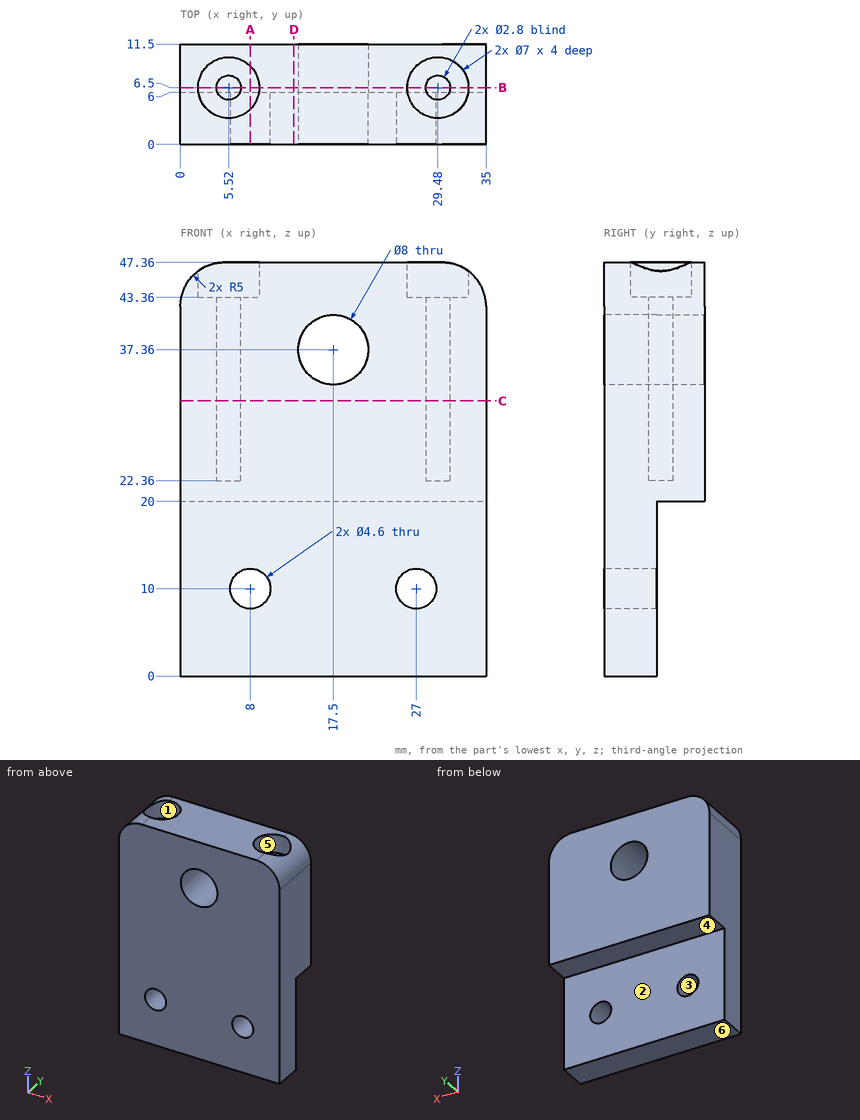
Geometry check sheet. Reference: drawing and pictorial views, mm from the part's lowest x, y, z. A direction names the side the tool comes from. Coordinates: 2 decimals unless noted, no trailing zeros. Write each loop counter-clockwise with the first axis right and the second up, starting at its lowest first coordinate (ties: lowest second). Pieces come first, ordered by that corner, then holes.
Item 1: Cross-section at D-D on x = 13. Record the boundary of the cut face in (y, z), then the cut area to 3 significant figures.
Numbers:
outline: (0, 0) - (6, 0) - (6, 20) - (11.5, 20) - (11.5, 47.36) - (0, 47.36) - close
area: 435 mm2
Item 2: Cross-section at A-A on x = 8. Record the boundary of the cut face in (y, z), then the cut area to 3 significant figures.
Numbers:
outline: (0, 0) - (6, 0) - (6, 7.7) - (0, 7.7) - close; (0, 12.3) - (6, 12.3) - (6, 20) - (11.5, 20) - (11.5, 47.36) - (8.97, 47.36) - (8.97, 43.36) - (4.03, 43.36) - (4.03, 47.36) - (0, 47.36) - close
area: 387 mm2
Item 3: Mould release check, pull along Y, two halves, no side actions. Record for the marked faces 1, 2 and 3: released by +Y, released by -Y, zero draft, split by the parting line, or undercut.
Numbers:
face 1: undercut
face 2: released by +Y
face 3: zero draft
Item 4: Cross-section at B-B on y = 6.5. Record the boundary of the cut face in (x, z) (1 decimal), then the cut area to 3 significant figures.
Numbers:
outline: (0, 20) - (35, 20) - (35, 42.4) arc R5 ccw to (33, 46.4) - (33, 43.4) - (30.9, 43.4) - (30.9, 22.4) - (28.1, 22.4) - (28.1, 43.4) - (26, 43.4) - (26, 47.4) - (9, 47.4) - (9, 43.4) - (6.9, 43.4) - (6.9, 22.4) - (4.1, 22.4) - (4.1, 43.4) - (2, 43.4) - (2, 46.4) arc R5 ccw to (0, 42.4) - close; hole circle Ø8 at (17.5, 37.4)
area: 725 mm2
Item 5: Depth check by flat-ended pin: pin 1 Ø2 at (x, y) = (29.5, 6) entering from +Z; pin 2 Ø1.7 at (x, y) = (5.52, 6.5) entering from +Z; pin 3 Ø6 at (x, y) = (24, 9.5) entering from -Z. Enter the tip coordinate at first touch or a pass-through.
Numbers:
pin 1: stops at z = 43.36
pin 2: stops at z = 22.36
pin 3: stops at z = 20
Item 6: Cross-section at C-C on z = 31.5. Record the boundary of the cut face in (x, y).
Numbers:
outline: (0, 0) - (35, 0) - (35, 11.5) - (0, 11.5) - close; hole circle Ø2.8 at (5.52, 6.5); hole circle Ø2.8 at (29.48, 6.5)
Item 7: Scan lines: probe 1 along Z at (x, y) = (27, 3.05); probe 2 along X at (y, z) = (2, 9); probe 3 along X at (y, z) = (3, 8.5). Record each from-to range of solid material in increasing order.
Numbers:
probe 1: z = 0 to 7.7, 12.3 to 47.36
probe 2: x = 0 to 5.93, 10.07 to 24.93, 29.07 to 35
probe 3: x = 0 to 6.26, 9.74 to 25.26, 28.74 to 35
Item 8: Access from +Z, -Z, +X, -X, +Y, -Y to the whole of each face (thin tool, end or side, straight path). Record for the marked faces 4, 5 and 6.
Numbers:
face 4: -Z, +X, -X, +Y
face 5: +Z
face 6: -Z, +X, -X, +Y, -Y
